Check sheet for the modelled part. Datum: model origin and axes. Units: mm. Coordinates: 2 decimals unless noted, no trailing zeros. Write each loop counter-clockwise with the first axis right and the second up, starting at its lowest first coordinate (ties: lowest second). Pieces come first, ordered by that corner, then holes. Notation, with made-up numbers: M -9.75,-15 L 35.25,-15 A22 ccw 35.25,-1 Z; hole C 32.25,31.5 d4. An arc over 180 degrees is marked long. Answer as CSV lines item,"result". Start each with the question number.
1) Section check B-B (z = 0.25). Record the cut outline in (x, y) (1 decimal), and give its area (3 significant figures).
2) Go/stop test with a flat-tipped pin: pin 1 Ø2 at (x, y) = (11.11, -8) entering from -Z. Record where the tip stops, or that it passes through.
3) Section check A-A (y = 8). Record the cut outline in (x, z) (3 decimals).
4) Draft check along X on faces 1 (the flat face through (0, 12.7, 0)), 2 (the cylindrical face through (-0.31, -6.89, 0.04)), 3 (the cylindrical face through (12.267, -7.521, 0.044)), 4 (the flat face through (22.225, 0, 0)). Enter one of: +X half, -X half, draft (parallel to the pull), parting line (faces both ways), or undercut.
5) Section check C-C (y = -7.5). Record the cut outline in (x, z) (3 decimals), and give its area (3 significant figures).
6) Material ranges on L1, parallel to X at y = -8, z = 1.75 (3 decimals); L2, parallel to Y at x = 10.5, z = 2.25; L3, parallel to X at y = 8.75, z = 0.75 (3 decimals), recorded low to high. Write a range as [from, to].
from build123d import *

# Parameters (mm, degrees)
ESQUISSE1_W             = 44.45
ESQUISSE1_H             = 25.4
BOSS_EXTRU_1_DEPTH      = 3.175
ESQUISSE2_R             = 1.24968
ENL_V_MAT_EXTRU_1_DEPTH = 27.373530765


with BuildPart() as part:
    # Esquisse1 → Boss.-Extru.1 (new, symmetric)
    with BuildSketch(Plane.XY):
        Rectangle(ESQUISSE1_W, ESQUISSE1_H)
    extrude(amount=BOSS_EXTRU_1_DEPTH, both=True)

    # Esquisse2 → Enlèv. mat.-Extru.1 (cut, through all)
    with BuildSketch(Plane.XY.offset(3.175)):
        with Locations((-0.8875, 8)):
            Circle(ESQUISSE2_R)
        with Locations((11.1125, 8)):
            Circle(ESQUISSE2_R)
    enl_v_mat_extru_1 = extrude(amount=-ENL_V_MAT_EXTRU_1_DEPTH, mode=Mode.SUBTRACT)

    # Symétrie1: Enlèv. mat.-Extru.1 across plane
    add(enl_v_mat_extru_1.mirror(Plane.ZX), mode=Mode.SUBTRACT)


solid = part.part
Results found:
1,outline,"M -22.2,-12.7 L 22.2,-12.7 L 22.2,12.7 L -22.2,12.7 Z; hole C -0.9,-8 d2.5; hole C -0.9,8 d2.5; hole C 11.1,-8 d2.5; hole C 11.1,8 d2.5"
1,area,"1,110 mm2"
2,pin 1,"passes through"
3,outline,"M -22.225,-3.175 L -2.137,-3.175 L -2.137,3.175 L -22.225,3.175 Z; M 0.362,-3.175 L 9.863,-3.175 L 9.863,3.175 L 0.362,3.175 Z; M 12.362,-3.175 L 22.225,-3.175 L 22.225,3.175 L 12.362,3.175 Z"
4,face 1,"draft"
4,face 2,"undercut"
4,face 3,"undercut"
4,face 4,"+X half"
5,outline,"M -22.225,-3.175 L -2.033,-3.175 L -2.033,3.175 L -22.225,3.175 Z; M 0.258,-3.175 L 9.967,-3.175 L 9.967,3.175 L 0.258,3.175 Z; M 12.258,-3.175 L 22.225,-3.175 L 22.225,3.175 L 12.258,3.175 Z"
5,area,"253 mm2"
6,L1,"x = [-22.225, -2.137], [0.362, 9.863], [12.362, 22.225]"
6,L2,"y = [-12.7, -9.09], [-6.91, 6.91], [9.09, 12.7]"
6,L3,"x = [-22.225, -1.887], [0.112, 10.113], [12.112, 22.225]"
